Autodesk Inventor part; units mm, degrees
ref_plane "YZ Plane" through (0, 0, 0) normal (1, 0, 0) x (0, 1, 0)
ref_plane "XZ Plane" through (0, 0, 0) normal (0, 1, 0) x (-1, 0, 0)
ref_plane "XY Plane" through (0, 0, 0) normal (0, 0, 1) x (1, 0, 0)
sketch "스케치1" plane through (0, 0, 0) normal (0, 0, 1) x (1, 0, 0)
  line L0 (-3, 0) -> (-1.5, 2.5981)
  line L1 (-1.5, 2.5981) -> (1.5, 2.5981)
  line L2 (1.5, 2.5981) -> (3, 0)
  line L3 (3, 0) -> (1.5, -2.5981)
  line L4 (1.5, -2.5981) -> (-1.5, -2.5981)
  line L5 (-1.5, -2.5981) -> (-3, 0)
  point P0 (0, 0)
  point P1 (0, 0)
  dimension "d0" = 6
extrude "돌출1" add sketch "스케치1" along normal blind 6
sketch "스케치2" plane through (0, 0, 6) normal (0, 0, 1) x (1, 0, 0)
  circle A0 centre (0, 0) radius 1.5
  dimension "d3" = 3
extrude "돌출2" add sketch "스케치2" along normal blind 5
sketch "스케치3" plane through (0, 0, 0) normal (0, 0, -1) x (-1, 0, 0)
  circle A0 centre (0, 0) radius 1.5
  dimension "d6" = 3
extrude "돌출3" cut sketch "스케치3" against normal blind 5
properties part number "50mm지지대"
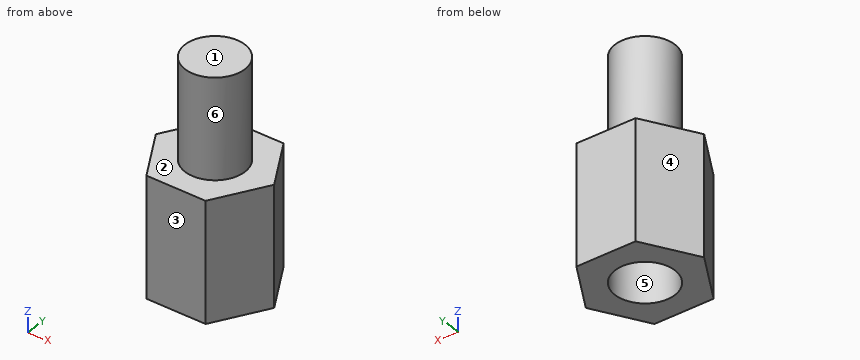
Can you work these out from the model? Positions are in its coordinate system, mm. Face numbers are marked on the shaded views. A direction names the side the tool comes from. Coordinates: 2 decimals unless noted, no trailing zeros. Order: outer loops, then holes, each group sorted by start corner. A loop starts at its lowest first (then second) coordinate and runs counter-clockwise, first axis right, second up. Notation, with made-up numbers: (30, 42) - (44, 42) arc R20 ccw to (44, 53) - close; hole circle Ø11 at (-7.5, 53). An arc over 180 degrees is marked (long way). Answer as a JSON object with one key per item and string values. Group by question number.
Q1. Imagine slicing it at D-D (z = 9.75). Please give me the cut outline in (x, y), and give its area (3 significant figures).
Q2. Will this pin go through, and if not, where does the flat tip stop? P1, Ø0.9, axis at x = 0.5, y = 0, coming from the -Z side.
Q3. On a 3-axis mill with a long thin cutter (end or side, diameter ignored), from which of +Z, -Z, +X, -X, +Y, -Y can I reach the whole of each face in a straight line? I mean the marked faces 1 and 2. Say none if no direction works.
Q4. Imagine slicing it at B-B (x = 0.45). Please give me the cut outline in (y, z).
Q5. I need wall thicknesses on line 1 (Y direction, x = 0, z = 2.3); line 2 (Z direction, x = 0.4, y = 0.25); line 3 (Z direction, x = -1.55, y = -0.05). Which ranges of each line are inside material? Lowest first, please. Write a range as from..to.
Q6. We'd pull the mould along Y, two halves only. Please class the marked faces 3, 4, 5 and 6: +Y half, -Y half, draft (parallel to the pull), parting line (faces both ways), or undercut.
Q7. Imagine slicing it at A-A (z = 2). Please give me the cut outline in (x, y).
Q8. Imagine slicing it at C-C (y = 0.75). Please give me the cut outline in (x, z), and give its area (3 significant figures).
Determined:
{
 "1": {"outline": "circle Ø3 at (0, 0)", "area": "7.07 mm2"},
 "2": {"P1": "stops at z = 5"},
 "3": {"face 1": "+Z, +X, -X, +Y, -Y", "face 2": "+Z"},
 "4": {"outline": "(-2.6, 0) - (-1.43, 0) - (-1.43, 5) - (1.43, 5) - (1.43, 0) - (2.6, 0) - (2.6, 6) - (1.43, 6) - (1.43, 11) - (-1.43, 11) - (-1.43, 6) - (-2.6, 6) - close"},
 "5": {"line 1": "y = -2.6..-1.5, 1.5..2.6", "line 2": "z = 5..11", "line 3": "z = 0..6"},
 "6": {"face 3": "-Y half", "face 4": "+Y half", "face 5": "undercut", "face 6": "parting line"},
 "7": {"outline": "(-3, 0) - (-1.5, -2.6) - (1.5, -2.6) - (3, 0) - (1.5, 2.6) - (-1.5, 2.6) - close; hole circle Ø3 at (0, 0)"},
 "8": {"outline": "(-2.57, 0) - (-1.3, 0) - (-1.3, 5) - (1.3, 5) - (1.3, 0) - (2.57, 0) - (2.57, 6) - (1.3, 6) - (1.3, 11) - (-1.3, 11) - (-1.3, 6) - (-2.57, 6) - close", "area": "30.8 mm2"}
}
